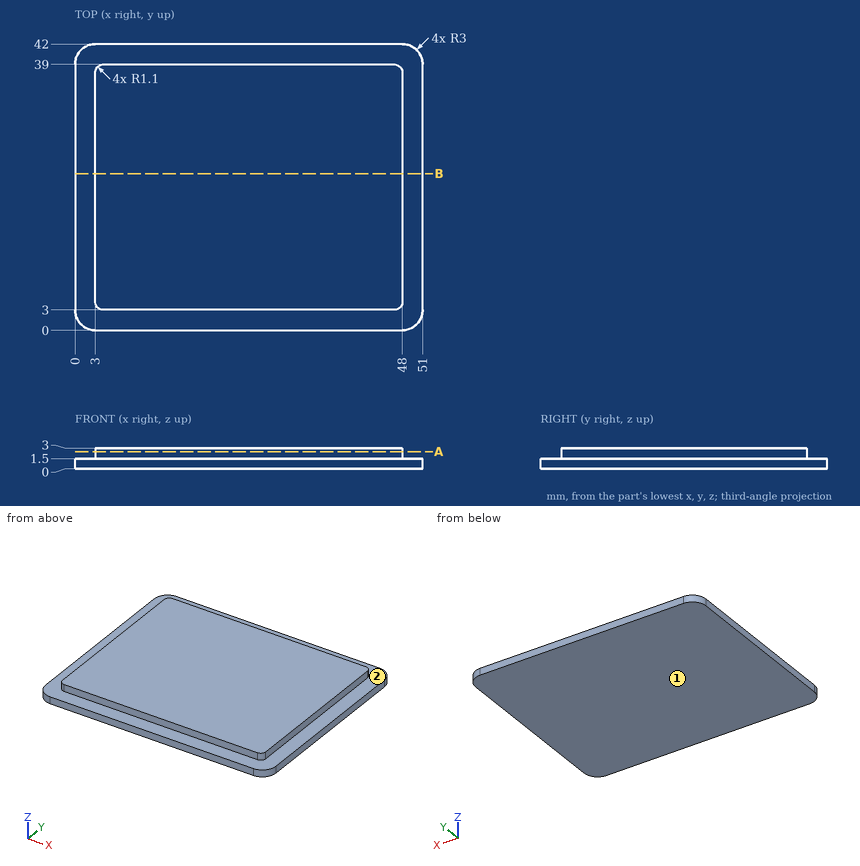
Design review of the part shown in the three views and the two pictorial views. Dimensions are in mm from the part's minimum x, y and z. A direction names the side the tool comes from. Round coordinates to 2 decimals unless told otherwise and drop trailing zeros. Order: outer loops, then holes, each group sorted by start corner. A loop starts at its lowest first (then second) coordinate and runs counter-clockwise, first axis right, second up. Notation, with made-up numbers: (-10, -36) - (42, -36) arc R19 ccw to (42, -12) - close; hole circle Ø7 at (84, 6.25). An arc over 180 degrees is marked (long way). One line per question, with ' | ' between items.
Item 1: Machinability: for the marked faces 1 and 2, which of the approach directions +Z, -Z, +X, -X, +Y, -Y give a long, thin tool a straight path to every point of the face, cutting with its end or side? Answer none if there is none.
Checks:
face 1: -Z, +X, -X, +Y, -Y | face 2: +Z
Item 2: Take a section at A-A, the plane z = 2.5. Write out the cut boundary in (x, y), then the cut area to 3 significant figures.
Checks:
outline: (3, 4.1) arc R1.1 ccw to (4.1, 3) - (46.9, 3) arc R1.1 ccw to (48, 4.1) - (48, 37.9) arc R1.1 ccw to (46.9, 39) - (4.1, 39) arc R1.1 ccw to (3, 37.9) - close | area: 1,620 mm²
Item 3: Take a section at B-B, the plane y = 23. Write out the cut boundary in (x, z).
Checks:
outline: (0, 0) - (51, 0) - (51, 1.5) - (48, 1.5) - (48, 3) - (3, 3) - (3, 1.5) - (0, 1.5) - close
Item 4: For P1, Ø0.8, axis at x = 33, z = 2.5, coming from the -Y side; P2, Ø0.8, axis at x = 33, z = 2.5, coming from the +Y side, all flat-tipped, find the tip position at first contact; note any pin that passes through.
Checks:
P1: y = 3 | P2: y = 39
Item 5: Wall thickness on line 1 (X direction, y = 12, z = 2.4); line 2 (Y direction, x = 25.5, z = 2.4); line 3 (X direction, y = 38.5, z = 2.25): over which ranges is each line inside the solid? List them lowest first. Write a range as [from, to].
Checks:
line 1: [3, 48] | line 2: [3, 39] | line 3: [3.18, 47.82]
